```python
from build123d import *

# Parameters (mm, degrees)
SM_BASE_FLANGE_1_DEPTH = 125


# Sheet-metal steps are written as plain solids
with BuildPart() as part:
    # Sketch 1 → 基体-法兰1 (new, symmetric)
    with BuildSketch(Plane.XY):
        with BuildLine():
            Line((-410, 0), (-220.414518843, 0))
            ThreePointArc((-220.414518843, 0), (-215.414518843, 1.339745962), (-211.754264805, 5))
            Line((-211.754264805, 5), (-185.773502692, 50))
            ThreePointArc((-185.773502692, 50), (-178.452994616, 57.320508076), (-168.452994616, 60))
            Line((-168.452994616, 60), (168.452994616, 60))
            ThreePointArc((168.452994616, 60), (178.452994616, 57.320508076), (185.773502692, 50))
            Line((185.773502692, 50), (211.754264805, 5))
            ThreePointArc((211.754264805, 5), (215.414518843, 1.339745962), (220.414518843, 0))
            Line((220.414518843, 0), (410, 0))
            Line((410, 0), (410, -10))
            Line((410, -10), (220.414518843, -10))
            ThreePointArc((220.414518843, -10), (210.414518843, -7.320508076), (203.094010768, 0))
            Line((203.094010768, 0), (177.113248654, 45))
            ThreePointArc((177.113248654, 45), (173.452994616, 48.660254038), (168.452994616, 50))
            Line((168.452994616, 50), (-168.452994616, 50))
            ThreePointArc((-168.452994616, 50), (-173.452994616, 48.660254038), (-177.113248654, 45))
            Line((-177.113248654, 45), (-203.094010768, 0))
            ThreePointArc((-203.094010768, 0), (-210.414518843, -7.320508076), (-220.414518843, -10))
            Line((-220.414518843, -10), (-410, -10))
            Line((-410, -10), (-410, 0))
        make_face()
    extrude(amount=SM_BASE_FLANGE_1_DEPTH, both=True)


solid = part.part
```
For this review, take the finished solid that the model builds, in its own axes (mm). A direction names the side the tool comes from. Coordinates: 2 decimals unless noted, no trailing zeros. Write each loop counter-clockwise with the first axis right and the second up, starting at its lowest first coordinate (ties: lowest second). Pieces come first, ordered by that corner, then holes. Notation, with made-up numbers: (-11.5, 37) - (11.5, 37) arc R15 ccw to (11.5, 44) - close; hole circle Ø7 at (3.5, -23.75). An arc over 180 degrees is marked (long way). Put each result on its own line as item: value.
1. Add section A-A, the plane y = 17. Give the boundary of the cut face in (x, z), then the cut area to 3 significant figures.
Values found:
outline: (-204.83, -125) - (-193.28, -125) - (-193.28, 125) - (-204.83, 125) - close; (193.28, -125) - (204.83, -125) - (204.83, 125) - (193.28, 125) - close
area: 5,770 mm²
2. Add section C-C, the plane x = -319. Give the boundary of the cut face in (y, z), then the cut area to 3 significant figures.
Values found:
outline: (-10, -125) - (0, -125) - (0, 125) - (-10, 125) - close
area: 2,500 mm²
3. Mouldability with a two-part tool opening along X and no side actions: class faces 4 (the flat face through (2, 54, 125)), 5 (the flat face through (190.29, 22.18, 1.75)), 6 (the flat face through (198.58, 27.82, 1.75)) as released by +X, released by -X, zero draft, split by the parting line, or undercut.
Values found:
face 4: zero draft
face 5: undercut
face 6: released by +X
4. For pin 1 (5 mm diameter, centred on y = 8, z = 81, fed in from -X); pin 2 (5 mm diameter, centred on x = -104, z = -99, fed in from -Y); pin 3 (12 mm diameter, centred on y = 28, z = -85.5, fed in from -X), all flat-tipped, find the tip position at first contact; note any pin that passes through.
Values found:
pin 1: x = -211.47
pin 2: y = 50
pin 3: x = -201.94
5. Add section B-B, the plane z = -18. Give the boundary of the cut face in (x, y).
Values found:
outline: (-410, -10) - (-220.41, -10) arc R20 ccw to (-203.09, 0) - (-177.11, 45) arc R10 cw to (-168.45, 50) - (168.45, 50) arc R10 cw to (177.11, 45) - (203.09, 0) arc R20 ccw to (220.41, -10) - (410, -10) - (410, 0) - (220.41, 0) arc R10 cw to (211.75, 5) - (185.77, 50) arc R20 ccw to (168.45, 60) - (-168.45, 60) arc R20 ccw to (-185.77, 50) - (-211.75, 5) arc R10 cw to (-220.41, 0) - (-410, 0) - close
6. Wall thickness on probe 1 along Y at (x, z) = (-376, -53); probe 2 along Y at (x, z) = (133, -25); probe 3 along X at (y, z) = (46, -0.5): over which ranges is each line inside the solid? List them lowest first.
Values found:
probe 1: -10 to 0
probe 2: 50 to 60
probe 3: -188.08 to -176.45, 176.45 to 188.08
7. Machinability: for faces 1 (the cylindrical face through (-210.29, -7.25, 1.75)), 2 (the flat face through (314, 0, 2)), 3 (the flat face through (-317, 0, 2)), which of the approach directions +Z, -Z, +X, -X, +Y, -Y give a long, thin tool a straight path to every point of the face, cutting with its end or side? Answer none if there is none.
Values found:
face 1: +Z, -Z, -Y
face 2: +Z, -Z, +X, +Y
face 3: +Z, -Z, -X, +Y
